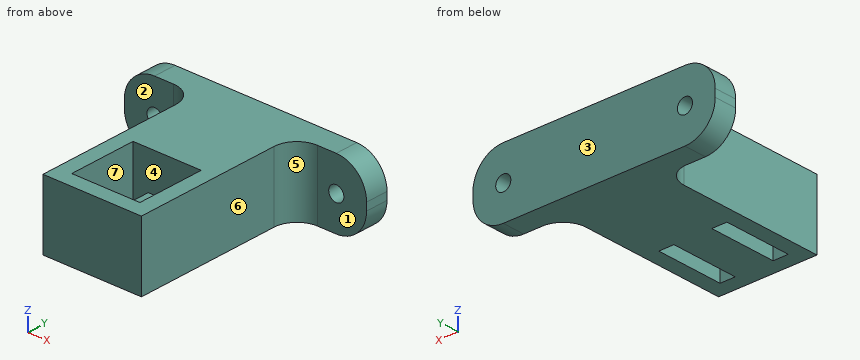
```python
from build123d import *

# Parameters (mm, degrees)
SKETCH1_W           = 13
SKETCH1_H           = 13
SKETCH1_W_2         = 5
SKETCH1_H_2         = 9
BOSS_EXTRUDE1_DEPTH = 4
SKETCH2_W           = 13
SKETCH2_H           = 13
SKETCH2_W_2         = 9
SKETCH2_H_2         = 9
BOSS_EXTRUDE2_DEPTH = 5
SKETCH3_W           = 13
SKETCH3_H           = 9
BOSS_EXTRUDE3_DEPTH = 12.5
BOSS_EXTRUDE4_DEPTH = 3
FILLET1_R           = 3
SKETCH5_R           = 1
CUT_EXTRUDE1_DEPTH  = 44.797830997


with BuildPart() as part:
    # Sketch1 → Boss-Extrude1 (new body)
    # profile 1 of 2: a face of its own
    with BuildSketch(Plane(origin=(0, 0, -30), x_dir=(-1, 0, 0), z_dir=(0, 0, -1))):
        with Locations((0, 6)):
            Rectangle(SKETCH1_W, SKETCH1_H)
        Polygon((-4.5, 10.5), (-2.5, 10.5), (2.5, 10.5), (4.5, 10.5), (4.5, 1.5), (2.5, 1.5), (-2.5, 1.5), (-4.5, 1.5), align=None, mode=Mode.SUBTRACT)
    # profile 2 of 2: a face of its own
    with BuildSketch(Plane(origin=(0, 0, -30), x_dir=(-1, 0, 0), z_dir=(0, 0, -1))):
        with Locations((0, 6)):
            Rectangle(SKETCH1_W_2, SKETCH1_H_2)
    extrude(amount=BOSS_EXTRUDE1_DEPTH)

    # Sketch2 → Boss-Extrude2 (add)
    with BuildSketch(Plane.XY.offset(-30)):
        with Locations((0, 6)):
            Rectangle(SKETCH2_W, SKETCH2_H)
        with Locations((0, 6)):
            Rectangle(SKETCH2_W_2, SKETCH2_H_2, mode=Mode.SUBTRACT)
    extrude(amount=BOSS_EXTRUDE2_DEPTH)

    # Sketch3 → Boss-Extrude3 (add)
    with BuildSketch(Plane(origin=(0, 12.5, 0), x_dir=(1, 0, 0), z_dir=(0, 1, 0))):
        with Locations((0, 29.5)):
            Rectangle(SKETCH3_W, SKETCH3_H)
    extrude(amount=BOSS_EXTRUDE3_DEPTH)

    # Sketch4 → Boss-Extrude4 (add)
    with BuildSketch(Plane(origin=(0, 25, 0), x_dir=(1, 0, 0), z_dir=(0, 1, 0))):
        with BuildLine():
            Line((-12, 25), (12, 25))
            ThreePointArc((12, 25), (14.828427125, 26.171572875), (16, 29))
            Line((16, 29), (16, 30))
            ThreePointArc((16, 30), (14.828427125, 32.828427125), (12, 34))
            Line((12, 34), (-12, 34))
            ThreePointArc((-12, 34), (-14.828427125, 32.828427125), (-16, 30))
            Line((-16, 30), (-16, 29))
            ThreePointArc((-16, 29), (-14.828427125, 26.171572875), (-12, 25))
        make_face()
    extrude(amount=-BOSS_EXTRUDE4_DEPTH)

    # Fillet1
    fillet1_edges = [part.edges().sort_by_distance(p)[0] for p in [
        (-6.5, 22, -29.5),
        (6.5, 22, -29.5),
    ]]
    fillet(fillet1_edges, radius=FILLET1_R)

    # Sketch5 → Cut-Extrude1 (cut, through all)
    with BuildSketch(Plane.XZ.offset(-22)):
        with Locations((-12, -29.5)):
            Circle(SKETCH5_R)
        with Locations((12, -29.5)):
            Circle(SKETCH5_R)
    extrude(amount=-CUT_EXTRUDE1_DEPTH, mode=Mode.SUBTRACT)


solid = part.part
```
Model file for the job. Use its own axes, mm. Face numbers are marked on the shaded views. A direction names the side the tool comes from. Give positions to 0.01 mm unless a question says otherwise; leave off trailing zeros. Order: outer loops, then holes, each group sorted by start corner. A loop starts at its lowest first (then second) coordinate and runs counter-clockwise, first axis right, second up.
1) Mould opens along Y. For the marked faces 5, 6 and 7 say: +Y half, -Y half, draft (parallel to the pull), parting line (faces both ways), or undercut.
2) Saw through at C-C, the plane y = 5.25. Write the cut outline in (x, z).
3) Pin check, flat tips, straight feed: pin 1 (3 mm diameter, centred on y = 8, z = -31, fed in from +X); pin 2 (2 mm diameter, centred on y = 7, z = -33, fed in from -X); pin 3 (12 mm diameter, centred on x = -3.5, y = 2.5, fed in from +Z); pin 4 (3 mm diameter, centred on x = -13.5, z = -29.5, fed in from -Y). Stop position of each tip, or through.
4) Wall check: probe 1 along Z at (x, y) = (-12, 24.3); probe 2 along X at (y, z) = (3.25, -26.75); probe 3 along X at (y, z) = (23, -29). Give the ranges that are in metal, low to high.
5) Saw through at D-D, the plane z = -33.5. Write the cut outline in (x, y), then the cut area to 3 significant figures.
6) 3-axis set-ups, long thin cutter, end or side, ignore diameter. For the marked faces 1, 2, 3 and 4: which of +Z, -Z, +X, -X, +Y, -Y reach the whole face in a straight line?
7) Saw through at B-B, the plane x = 3. Write the cut outline in (y, z), then the cut area to 4 significant figures.
8) Saw through at A-A, the plane z = -29.5. Write the cut outline in (x, y).
Computed:
1. face 5: -Y half
1. face 6: draft
1. face 7: undercut
2. outline: (-6.5, -34) - (-4.5, -34) - (-4.5, -25) - (-6.5, -25) - close; (-2.5, -34) - (2.5, -34) - (2.5, -30) - (-2.5, -30) - close; (4.5, -34) - (6.5, -34) - (6.5, -25) - (4.5, -25) - close
3. pin 1: stops at x = 6.5
3. pin 2: stops at x = -6.5
3. pin 3: stops at z = -25
3. pin 4: stops at y = 22
4. probe 1: z = -34 to -30.5, -28.5 to -25
4. probe 2: x = -6.5 to -4.5, 4.5 to 6.5
4. probe 3: x = -16 to -12.87, -11.13 to 11.13, 12.87 to 16
5. outline: (-13.94, 22) - (-9.5, 22) arc R3 cw to (-6.5, 19) - (-6.5, -0.5) - (6.5, -0.5) - (6.5, 19) arc R3 cw to (9.5, 22) - (13.94, 22) - (13.94, 25) - (-13.94, 25) - close; hole (-4.5, 1.5) - (-2.5, 1.5) - (-2.5, 10.5) - (-4.5, 10.5) - close; hole (2.5, 1.5) - (4.5, 1.5) - (4.5, 10.5) - (2.5, 10.5) - close
5. area: 344 mm2
6. face 1: +Z, -Z, +X, -Y
6. face 2: +Z, -Z, -X, -Y
6. face 3: +Z, -Z, +X, -X, +Y
6. face 4: +Z
7. outline: (-0.5, -34) - (1.5, -34) - (1.5, -25) - (-0.5, -25) - close; (10.5, -34) - (25, -34) - (25, -25) - (10.5, -25) - close
7. area: 148.5 mm2
8. outline: (-16, 22) - (-13, 22) - (-13, 25) - (-16, 25) - close; (-11, 22) - (-9.5, 22) arc R3 cw to (-6.5, 19) - (-6.5, -0.5) - (6.5, -0.5) - (6.5, 19) arc R3 cw to (9.5, 22) - (11, 22) - (11, 25) - (-11, 25) - close; (13, 22) - (16, 22) - (16, 25) - (13, 25) - close; hole (-4.5, 1.5) - (4.5, 1.5) - (4.5, 10.5) - (-4.5, 10.5) - close
